Work out the finished part from the listing and answer in its coordinate system (mm). A direction names the side the tool comes from. Coordinates: 2 decimals unless noted, no trailing zeros. Order: outer loops, then holes, each group sorted by start corner. A loop starts at its lowest first (then second) coordinate and runs counter-clockwise, first axis right, second up. Notation, with made-up numbers: M -12,-23 L -6,-23 A14 ccw -6,-18 Z; hole C -37.5,-27.75 d7. An arc over 180 degrees is marked long. Use a Markdown table: item, result.
Autodesk Inventor part; units mm, degrees
ref_plane "YZ Plane" through (0, 0, 0) normal (1, 0, 0) x (0, 1, 0)
ref_plane "XZ Plane" through (0, 0, 0) normal (0, 1, 0) x (-1, 0, 0)
ref_plane "XY Plane" through (0, 0, 0) normal (0, 0, 1) x (1, 0, 0)
sketch "Sketch1" plane through (0, 0, 0) normal (0, 0, 1) x (1, 0, 0)
  line L0 (-14.4256, 5.5876) -> (8.1894, 5.5876)
  line L1 (8.1894, 5.5876) -> (8.1894, 11.7876)
  line L2 (8.1894, 11.7876) -> (34.7894, 11.7876)
  line L3 (34.7894, 11.7876) -> (34.7894, 5.5876)
  line L4 (34.7894, 5.5876) -> (57.4044, 5.5876)
  line L5 (57.4044, 5.5876) -> (57.4044, -0.6124)
  line L6 (57.4044, -0.6124) -> (34.4294, -0.6124)
  line L7 (-14.4256, 5.5876) -> (-14.4256, -0.6124)
  line L8 (-14.4256, -0.6124) -> (8.5494, -0.6124)
  line L9 (21.4894, 2.3876) -> (8.5494, -0.6124)
  line L10 (21.4894, 2.3876) -> (34.4294, -0.6124)
  point P0 (0, 0)
  dimension "d0" = 22.615
  dimension "d1" = 6.2
  dimension "d2" = 26.6
  dimension "d3" = 22.615
  dimension "d4" = 6.2
  dimension "d5" = 22.975
  dimension "d9" = 22.975
extrude "Extrusion1" add sketch "Sketch1" against normal blind 12.64
sketch "Sketch2" plane through (-14.4256, 5.5876, 0) normal (0, 1, 0) x (1, 0, 0)
  circle A0 centre (11.488, 6.46) radius 3.175
  circle A1 centre (60.342, 6.46) radius 3.175
  line L0 (0, 0) -> (0, 12.64)
  line L1 (0, 12.64) -> (22.615, 12.64)
  line L2 (49.215, 12.64) -> (71.83, 12.64)
  line L3 (71.83, 0) -> (71.83, 12.64)
  point P0 (14.4256, 0)
  dimension "d14" = 11.488
  dimension "d15" = 6.18
  dimension "d16" = 6.35
  dimension "d17" = 6.18
  dimension "d18" = 11.488
  dimension "d19" = 6.35
extrude "Extrusion2" cut sketch "Sketch2" against normal blind 12.64
thread "Thread1"
thread "Thread2"
properties part number "syringe holder"
(1) A cutting plane is placed at C-C (y = 1.25). Determine the outline of the cut face in (x, z) (3 decimals).
Conclusion:
| item | result |
|---|---|
| outline | M -14.426,-12.64 L 16.583,-12.64 L 16.583,0 L -14.426,0 Z; M 26.396,-12.64 L 57.404,-12.64 L 57.404,0 L 26.396,0 Z; hole C -2.938,-6.46 d6.35; hole C 45.916,-6.46 d6.35 |
(2) Which of the six approach directions +Z, -Z, +X, -X, +Y, -Y give full straight-line access (tool end or side, diameter ignored) to faces 1 (the flat face through (-6, -0.612, -9)), 2 (the flat face through (15.11, 0.91, -6.23)), 3 (the flat face through (43, 5.588, -9)), 4 (the flat face through (8.189, 9, -6))?
Conclusion:
| item | result |
|---|---|
| face 1 | +Z, -Z, +X, -X, -Y |
| face 2 | +Z, -Z, -Y |
| face 3 | +Z, -Z, +X, +Y |
| face 4 | +Z, -Z, -X, +Y |
(3) Given P1, Ø2, axis at x = -5.5, y = 7.5, coming from the +Z side; P2, Ø4, axis at x = 48.5, z = -6.5, coming from the +Y side; P3, Ø1, axis at x = 22.5, z = -4, coming from the -Y side; P4, Ø1.9, axis at y = 8, z = -3.5, coming from the +X side, each flat-ended and moving along its own axis, determine where each tip first touches the part or whether it passes through.
Conclusion:
| item | result |
|---|---|
| P1 | through |
| P2 | y = 5.59 |
| P3 | y = 2.04 |
| P4 | x = 34.79 |
(4) Determine the mould class of faces 5 (the flat face through (21, 4, 0)), 6 (the flat face through (-14.426, 3, -6)), 7 (the cylindrical face through (48.849, 2.531, -5.244)) for opening direction Z: pulls with the +Z half, pulls with the -Z half, needs draft (parallel to the pull), parting line crosses it, or undercut.
Conclusion:
| item | result |
|---|---|
| face 5 | pulls with the +Z half |
| face 6 | needs draft |
| face 7 | undercut |
(5) A cutting plane is placed at A-A (z = -6.46). Determine the outline of the cut face in (x, y).
Conclusion:
| item | result |
|---|---|
| outline | M -14.43,-0.61 L -6.11,-0.61 L -6.11,5.59 L -14.43,5.59 Z; M 0.24,-0.61 L 8.55,-0.61 L 21.49,2.39 L 34.43,-0.61 L 42.74,-0.61 L 42.74,5.59 L 34.79,5.59 L 34.79,11.79 L 8.19,11.79 L 8.19,5.59 L 0.24,5.59 Z; M 49.09,-0.61 L 57.4,-0.61 L 57.4,5.59 L 49.09,5.59 Z |
(6) A cutting plane is placed at B-B (x = 45.5). Determine the outline of the cut face in (y, z).
Conclusion:
| item | result |
|---|---|
| outline | M -0.61,-12.64 L 5.59,-12.64 L 5.59,-9.61 L -0.61,-9.61 Z; M -0.61,-3.31 L 5.59,-3.31 L 5.59,0 L -0.61,0 Z |
(7) A cutting plane is placed at D-D (z = -11.25). Determine the outline of the cut face in (x, y), then the cut area to 3 significant figures.
Conclusion:
| item | result |
|---|---|
| outline | M -14.43,-0.61 L 8.55,-0.61 L 21.49,2.39 L 34.43,-0.61 L 57.4,-0.61 L 57.4,5.59 L 34.79,5.59 L 34.79,11.79 L 8.19,11.79 L 8.19,5.59 L -14.43,5.59 Z |
| area | 571 mm2 |
(8) Straight lines are drawn through the part: L1, parallel to X at y = 3.25, z = -6.46; L2, parallel to Y at x = 44, z = -2.5; L3, parallel to X at y = 7.5, z = -6.75. For each, find the intervals that lie inside material, in ascending order.
Conclusion:
| item | result |
|---|---|
| L1 | -14.43 to -6.11, 0.24 to 42.74, 49.09 to 57.4 |
| L2 | -0.61 to 5.59 |
| L3 | 8.19 to 34.79 |
